Geometry: final body of the model. Coordinates: model frame, mm. Give positions to 0.01 mm unless a question says otherwise; leave off trailing zeros. Loops run counter-clockwise (first coordinate to the right, second up) from the corner with the lowest first, then second, coordinate; pieces in that order, holes last. Notation, with made-up numbers: (58, 71.5) -> (108, 71.5) arc R26 ccw to (108, 95.5) -> close; hole circle Ø1 at (39, 67). An arc over 180 degrees is marked (long way). Answer in a Markdown table with one row per item. Add a question column.
1) First-contact query: P1, Ø2, axis at y = 1, z = -0.5, coming from the +X side; P2, Ø1.4, axis at x = 0.5, z = -0.5, coming from the -Y side. Flat tips, straight axial feed; report the tip coordinate or a pass-through.
2) Section query C-C (y = 1.75). Return the cut outline in (x, z) (3 decimals).
3) Draft query along Z for faces 1 (the cylindrical face through (3, 3, 0)), 2 (the flat face through (0, 1, 1.375)), 3 (the flat face through (0, 8, 0)). Return one class per face: +Z half, -Z half, draft (parallel to the pull), parting line (faces both ways), or undercut.
4) Section query B-B (x = 0). Return the cut outline in (y, z) (3 decimals), plus the area to 3 significant figures.
5) Line query: line 1 (Y direction, x = 1, z = -0.25); line 2 (Y direction, x = -1.8, z = -1); line 3 (X direction, y = 5.25, z = 0.5). Output: solid intervals per line, ascending. Write a range as from..to.
6) Section query D-D (y = 6). Return the cut outline in (x, z).
7) Section query A-A (z = 0). Return the cut outline in (x, y) (3 decimals).
Autodesk Inventor part; units mm, degrees
ref_plane "YZ Plane" through (0, 0, 0) normal (1, 0, 0) x (0, 1, 0)
ref_plane "XZ Plane" through (0, 0, 0) normal (0, 1, 0) x (-1, 0, 0)
ref_plane "XY Plane" through (0, 0, 0) normal (0, 0, 1) x (1, 0, 0)
sketch "Sketch1" plane through (0, 0, 0) normal (0, 1, 0) x (-1, 0, 0)
  circle A0 centre (0, 0) radius 3
  dimension "d0" = 6
extrude "Extrusion1" add sketch "Sketch1" along normal blind 8
sketch "Sketch2" plane through (0, 0, 0) normal (0, -1, 0) x (1, 0, 0)
  line L0 (-1.375, -1.375) -> (1.375, -1.375)
  line L1 (1.375, -1.375) -> (1.375, 1.375)
  line L2 (1.375, 1.375) -> (-1.375, 1.375)
  line L3 (-1.375, 1.375) -> (-1.375, -1.375)
  line L4 (-1.375, -1.375) -> (1.375, 1.375) construction
  line L5 (1.375, -1.375) -> (-1.375, 1.375) construction
  point P0 (0, 0)
  dimension "d3" = 2.75
  dimension "d4" = 2.75
extrude "Extrusion2" cut sketch "Sketch2" against normal blind 2.5
fillet "Fillet1" radius 1 1 edges at (3, 8, 0)
properties part number "Button"
Evaluation:
| question | item | result |
|---|---|---|
| 1 | P1 | x = 3 |
| 1 | P2 | y = 2.5 |
| 2 | outline | circle Ø6 at (0, 0); hole (-1.375, -1.375) -> (1.375, -1.375) -> (1.375, 1.375) -> (-1.375, 1.375) -> close |
| 3 | face 1 | parting line |
| 3 | face 2 | undercut |
| 3 | face 3 | draft |
| 4 | outline | (0, -3) -> (7, -3) arc R1 ccw to (8, -2) -> (8, 2) arc R1 ccw to (7, 3) -> (0, 3) -> (0, 1.375) -> (2.5, 1.375) -> (2.5, -1.375) -> (0, -1.375) -> close |
| 4 | area | 40.7 mm² |
| 5 | line 1 | 2.5..8 |
| 5 | line 2 | 0..8 |
| 5 | line 3 | -2.96..2.96 |
| 6 | outline | circle Ø6 at (0, 0) |
| 7 | outline | (-3, 0) -> (-1.375, 0) -> (-1.375, 2.5) -> (1.375, 2.5) -> (1.375, 0) -> (3, 0) -> (3, 7) arc R1 ccw to (2, 8) -> (-2, 8) arc R1 ccw to (-3, 7) -> close |
